```python
from build123d import *

# Parameters (mm, degrees)
SKETCH1_R                                          = 14.2875
BOSS_EXTRUDE1_DEPTH                                = 3.175
F_6_CLEARANCE_HOLE3_D                              = 4.3053
CUT_EXTRUDE1_DEPTH                                 = 255.792513626
CHAMFER1_SIZE                                      = 3.81
CSK_FOR_6_FLAT_HEAD_MACHINE_SCREW_100_D            = 4.3053
CSK_FOR_6_FLAT_HEAD_MACHINE_SCREW_100_CSINK_D      = 7.0866
CSK_FOR_6_FLAT_HEAD_MACHINE_SCREW_100_CSINK_ANGLE  = 100
SKETCH14_W                                         = 50.8
SKETCH14_H                                         = 38.1
BOSS_EXTRUDE2_DEPTH                                = 6.35
CHAMFER2_SIZE                                      = 2.54
CSK_FOR_10_FLAT_HEAD_MACHINE_SCREW_100_D           = 5.6134
CSK_FOR_10_FLAT_HEAD_MACHINE_SCREW_100_CSINK_D     = 9.779
CSK_FOR_10_FLAT_HEAD_MACHINE_SCREW_100_CSINK_ANGLE = 100
F_1_4_0_25_DIAMETER_HOLE1_D                        = 6.35
F_15_32_0_46875_DIAMETER_HOLE1_D                   = 11.90625


with BuildPart() as part:
    # Sketch1 → Boss-Extrude1 (new, symmetric)
    with BuildSketch(Plane.XY):
        Polygon((0, 19.05), (-28.575, 19.05), (-28.575, -19.05), (0, -19.05), (247.281942035, -19.05), (254, 19.05), align=None)
        Circle(SKETCH1_R, mode=Mode.SUBTRACT)
    extrude(amount=BOSS_EXTRUDE1_DEPTH, both=True)

    # #6 Clearance Hole3 (through all)
    with Locations(Plane.XY.offset(3.175)):
        with Locations((229.388701471, 8.923791784), (229.282371239, -11.346798968), (203.503161764, -11.143926969), (203.608782335, 8.991375351), (165.672159691, 8.991375351), (165.672159691, -11.143926969), (151.067159691, 0)):
            Hole(F_6_CLEARANCE_HOLE3_D / 2)

    # Sketch9 → Cut-Extrude1 (cut, through all)
    with BuildSketch(Plane.XY.offset(3.175)):
        Polygon((254, 19.05), (247.281942035, -19.05), (237.352085197, -19.05), (237.352085197, 19.05), align=None)
    extrude(amount=-CUT_EXTRUDE1_DEPTH, mode=Mode.SUBTRACT)

    # Chamfer1
    chamfer1_edges = [part.edges().sort_by_distance(p)[0] for p in [
        (-28.575, -19.05, 0),
        (-28.575, 19.05, 0),
        (237.352085197, 19.05, 0),
        (237.352085197, -19.05, 0),
    ]]
    chamfer(chamfer1_edges, length=CHAMFER1_SIZE)

    # CSK for #6 Flat Head Machine Screw (100)2 (through all)
    with Locations(Plane.XY.offset(3.175)):
        with Locations((203.608782335, 8.991375351), (203.503161764, -11.143926969), (229.282371239, -11.346798968), (229.388701471, 8.923791784), (165.672159691, 8.991375351), (165.672159691, -11.143926969), (151.067159691, 0)):
            CounterSinkHole(CSK_FOR_6_FLAT_HEAD_MACHINE_SCREW_100_D / 2, CSK_FOR_6_FLAT_HEAD_MACHINE_SCREW_100_CSINK_D / 2, counter_sink_angle=CSK_FOR_6_FLAT_HEAD_MACHINE_SCREW_100_CSINK_ANGLE)

    # Sketch14 → Boss-Extrude2 (add, through all)
    with BuildSketch(Plane.XY.offset(3.175)):
        with Locations((-50.165, 0)):
            Rectangle(SKETCH14_W, SKETCH14_H)
    extrude(amount=-BOSS_EXTRUDE2_DEPTH)

    # Chamfer2
    chamfer2_edges = [part.edges().sort_by_distance(p)[0] for p in [
        (-75.565, -19.05, 0),
        (-75.565, 19.05, 0),
    ]]
    chamfer(chamfer2_edges, length=CHAMFER2_SIZE)

    # CSK for #10 Flat Head Machine Screw (100)1 (through all)
    with Locations(Plane(origin=(0, 0, -3.175), x_dir=(1, 0, 0), z_dir=(0, 0, -1))):
        with Locations((-65.405, 0)):
            CounterSinkHole(CSK_FOR_10_FLAT_HEAD_MACHINE_SCREW_100_D / 2, CSK_FOR_10_FLAT_HEAD_MACHINE_SCREW_100_CSINK_D / 2, counter_sink_angle=CSK_FOR_10_FLAT_HEAD_MACHINE_SCREW_100_CSINK_ANGLE)

    # 1/4 (0.25) Diameter Hole1 (through all)
    with Locations(Plane(origin=(0, 0, -3.175), x_dir=(-1, 0, 0), z_dir=(0, 0, -1))):
        with Locations((33.655, 0)):
            Hole(F_1_4_0_25_DIAMETER_HOLE1_D / 2)

    # 15/32 (0.46875) Diameter Hole1 (through all)
    with Locations(Plane(origin=(0, 0, -3.175), x_dir=(-1, 0, 0), z_dir=(0, 0, -1))):
        with Locations((-93.967218212, 0)):
            Hole(F_15_32_0_46875_DIAMETER_HOLE1_D / 2)


solid = part.part
```
Geometry check sheet. Reference: the model listing, model coordinates, mm. Round coordinates to 2 decimals unless told otherwise and drop trailing zeros. Return JSON: item names as keys, results as strings. Group by question number.
(1) Go/stop test with a flat-tipped pin: pin 1 (6.5 mm diameter, centred on x = -65.405, y = 0, fed in from -Z). Record where the tip stops, or that it passes through.
(2) Mould release check, pull along X, two halves, no side actions. Record for faces 1 (the face through (-62.6, -0.1, 0.9)), 2 (the face through (-75.565, 0, 0)), 3 (the face through (237.352, 0, 0)), 4 (the face through (79, 0, 3.175)): pulls with the +X half, pulls with the -X half, needs draft (parallel to the pull), parting line crosses it, or undercut.
(3) Section check B-B, the plane z = -0.25. Give the number of separate pieces and of enclosed holes in the cut face, and give its area (3 significant figures).
(4) Scan lines: line 1 along X through (y, z) = (13, -1.5) (3 decimals); line 2 along X through (y, z) = (-11.5, 2.25) (3 decimals); line 3 along Y through (x, z) = (-0.5, -1). Record each from-to range of solid material in increasing order. Write a range as [from, to].
Data:
{
 "1": {"pin 1": "z = -1.8"},
 "2": {"face 1": "undercut", "face 2": "pulls with the -X half", "face 3": "pulls with the +X half", "face 4": "needs draft"},
 "3": {"separate pieces": "1", "enclosed holes": "11", "area": "11,000 mm²"},
 "4": {"line 1": "[-75.565, -5.927], [5.927, 237.352]", "line 2": "[-75.565, -8.478], [8.478, 163.257], [168.087, 201.088], [205.918, 226.846], [231.718, 237.352]", "line 3": "[-19.05, -14.28], [14.28, 19.05]"}
}
